Verification items for the finished model (mm, model axes). Face numbers are marked on the shaded views. A direction names the side the tool comes from. Round coordinates to 2 decimals unless told otherwise and drop trailing zeros. Order: outer loops, then holes, each group sorted by start corner. A loop starts at its lowest first (then second) coordinate and runs counter-clockwise, first axis right, second up. Notation, with made-up numbers: (-7.5, 2.5) -> (2.5, 2.5) arc R16 cw to (2.5, 33.5) -> close; hole circle Ø7 at (64, 0.25). An arc over 180 degrees is marked (long way). Return JSON: item names as keys, results as strings. Group by question number.
1) Section check B-B on x = 195.5. Enter the section's corners in (y, z).
2) Tool access check on the marked faces 1, 2 and 3. Record the directions out of +Z, -Z, +X, -X, +Y, -Y that give a thin tool (end or side, any length) a straight path to the whole face; none if there is none.
3) Depth check by flat-ended pin: pin 1 (24 mm diameter, centred on x = -17.5, y = 15.5, fed in from -Z); pin 2 (11 mm diameter, centred on x = -12.5, z = 2, fed in from +Y); pin 3 (1.5 mm diameter, centred on x = 202.5, y = 23.5, fed in from -Z). Enter the tip coordinate at first touch or a pass-through.
4) Section check C-C on z = 21.5. Enter the section's corners in (x, y), plus the area to 3 significant figures.
5) Section check A-A on z = 0. Enter the section's corners in (x, y), plus the area to 3 significant figures.
6) Scan lines: L1, parallel to X at y = 8, z = -7.5; L2, parallel to X at y = -7, z = -4; L3, parallel to Y at x = 63, z = -1. Record each from-to range of solid material in increasing order.
7) Section check D-D on z = -19.5. Enter the section's corners in (x, y), plus the area to 3 significant figures.
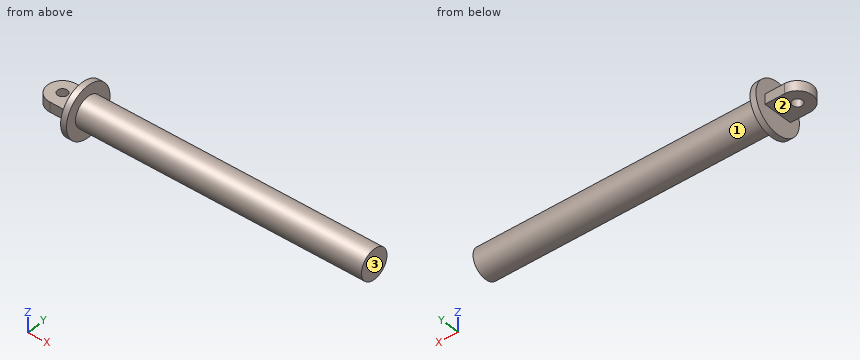
```python
from build123d import *

# Parameters (mm, degrees)
SKETCH2_R           = 5
BOSS_EXTRUDE1_DEPTH = 5


with BuildPart() as part:
    # Sketch2 → Boss-Extrude1 (new, symmetric)
    with BuildSketch(Plane.XY):
        with BuildLine():
            Line((-25.982341551, 28.402024397), (-5.982341551, 28.402024397))
            Line((-5.982341551, 28.402024397), (-5.982341551, -1.597975603))
            Line((-5.982341551, -1.597975603), (-25.982341551, -1.597975603))
            ThreePointArc((-25.982341551, -1.597975603), (-40.982341551, 13.402024397), (-25.982341551, 28.402024397))
        make_face()
        with Locations((-25.982341551, 13.402024397)):
            Circle(SKETCH2_R, mode=Mode.SUBTRACT)
    extrude(amount=BOSS_EXTRUDE1_DEPTH, both=True)

    # Sketch8 → Revolve1 (revolve)
    with BuildSketch(Plane.XY):
        Polygon((-5.982341551, 28.402024397), (-5.982341551, 39), (0, 39), (0, 28.402024397), (289.215653405, 28.402024397), (289.215653405, 13.402024397), (-5.982341551, 13.402024397), align=None)
    revolve(axis=Axis((289.215653405, 13.402024397, 0), (-1, 0, 0)))


solid = part.part
```
Check result:
{
 "1": {"outline": "circle Ø30 at (13.4, 0)"},
 "2": {"face 1": "+X", "face 2": "-Z, -X, +Y, -Y", "face 3": "+Z, -Z, +X, +Y, -Y"},
 "3": {"pin 1": "z = -25.6", "pin 2": "y = 28.4", "pin 3": "z = -11.73"},
 "4": {"outline": "(-5.98, -0.49) -> (0, -0.49) -> (0, 27.29) -> (-5.98, 27.29) -> close", "area": "166 mm^2"},
 "5": {"outline": "(-25.98, -1.6) -> (-5.98, -1.6) -> (-5.98, -12.2) -> (0, -12.2) -> (0, -1.6) -> (289.22, -1.6) -> (289.22, 28.4) -> (0, 28.4) -> (0, 39) -> (-5.98, 39) -> (-5.98, 28.4) -> (-25.98, 28.4) arc R15 ccw to start; hole circle Ø10 at (-25.98, 13.4)", "area": "9,860 mm^2"},
 "6": {"L1": "-5.98 to 289.22", "L2": "-5.98 to 0", "L3": "-1.56 to 28.37"},
 "7": {"outline": "(-5.98, -3.18) -> (0, -3.18) -> (0, 29.99) -> (-5.98, 29.99) -> close", "area": "198 mm^2"}
}
